Autodesk Inventor part; units mm, degrees
ref_plane "YZ Plane" through (0, 0, 0) normal (1, 0, 0) x (0, 1, 0)
ref_plane "XZ Plane" through (0, 0, 0) normal (0, 1, 0) x (-1, 0, 0)
ref_plane "XY Plane" through (0, 0, 0) normal (0, 0, 1) x (1, 0, 0)
sketch "Sketch1" plane through (0, 0, 0) normal (0, 0, 1) x (1, 0, 0)
  line L0 (0, 0) -> (0, 25.4)
  line L1 (0, 0) -> (25.4, 0)
  line L2 (4.7625, 20.6375) -> (4.7625, 9.525)
  line L3 (9.525, 4.7625) -> (20.6375, 4.7625)
  arc A0 (4.7625, 20.6375) -> (0, 25.4) centre (0, 20.6375) ccw
  arc A1 (25.4, 0) -> (20.6375, 4.7625) centre (20.6375, 0) ccw
  arc A2 (4.7625, 9.525) -> (9.525, 4.7625) centre (9.525, 9.525) ccw
  dimension "d0" = 25.4
  dimension "d1" = 25.4
  dimension "d2" = 4.7625
  dimension "d3" = 4.7625
extrude "Extrusion1" add sketch "Sketch1" along normal blind 25.4
sketch "Sketch2" plane through (0, 0, 0) normal (0, -1, 0) x (1, 0, 0)
  line L0 (25.4, 25.4) -> (0, 25.4)
  line L1 (25.4, 0) -> (25.4, 25.4)
  circle A0 centre (12.7, 12.7) radius 3.175
  dimension "d6" = 6.35
  dimension "d7" = 12.7
  dimension "d8" = 12.7
extrude "Extrusion2" cut sketch "Sketch2" against normal blind 25.4
sketch "Sketch3" plane through (0, 0, 0) normal (-1, 0, 0) x (0, 0, 1)
  circle A0 centre (12.7, 12.7) radius 3.175
  dimension "d11" = 6.35
extrude "Extrusion3" cut sketch "Sketch3" against normal blind 25.4
equation "\"d3\" = d2"
properties part number "small L bracket"
The model under review builds one solid part; all positions refer to its coordinate system, in mm. A direction names the side the tool comes from. Coordinates: 2 decimals unless noted, no trailing zeros. Write each loop counter-clockwise with the first axis right and the second up, starting at its lowest first coordinate (ties: lowest second). Pieces come first, ordered by that corner, then holes.
1) We need section A-A on y = 12.7. State the section outline as (x, z) points (1 decimal), then the cut area to 3 significant figures.
2) We need section D-D on x = 3. State the section outline as (y, z) points (3 decimals), then the cut area to 3 significant figures.
3) Machinability: for faces 4 (the face through (10.18, 2.35, 10.77)), 5 (the face through (16.2, 4.762, 12.5)), which of the approach directions +Z, -Z, +X, -X, +Y, -Y give a long, thin tool a straight path to every point of the face, cutting with its end or side? Answer none if there is none.
4) We need section C-C on z = 8.5. State the section outline as (x, y) points (1 decimal), then the cut area to 3 significant figures.
5) The part is to be moulded in two halves that separate along Z. For faces 1 (the face through (0, 15.3, 15.3)), 2 (the face through (2.35, 10.77, 10.18)), 3 (the face through (4, 7, 25.4)), say which applies: pulls with the +Z half, pulls with the -Z half, needs draft (parallel to the pull), parting line crosses it, or undercut.
6) To check wall thickness, follow probe 1 along Z at (x, y) = (1.75, 12.7) (3 decimals); probe 2 along Y at (x, z) = (20, 11). State the ranges of each line that lie inside material, in increasing order.
7) Clearance check with flat-ended pins moving along their axes: pin 1 Ø5 at (x, z) = (9, 14.5) entering from +Y; pin 2 Ø12 at (y, z) = (15, 14.5) entering from +X; pin 3 Ø5 at (x, z) = (12.7, 12.7) entering from +Y; pin 4 Ø12 at (x, z) = (13, 17.5) entering from +Y. State where each tip first meets the part, or that it passes through.
Answer list:
1. outline: (0, 0) - (4.8, 0) - (4.8, 9.5) - (0, 9.5) - close; (0, 15.9) - (4.8, 15.9) - (4.8, 25.4) - (0, 25.4) - close
1. area: 90.7 mm2
2. outline: (0, 0) - (24.336, 0) - (24.336, 25.4) - (0, 25.4) - close; hole circle Ø6.35 at (12.7, 12.7)
2. area: 586 mm2
3. face 4: +Y, -Y
3. face 5: +Z, -Z, +X, +Y
4. outline: (0, 0) - (25.4, 0) arc R4.8 ccw to (20.6, 4.8) - (9.5, 4.8) arc R4.8 cw to (4.8, 9.5) - (4.8, 20.6) arc R4.8 ccw to (0, 25.4) - close
4. area: 214 mm2
5. face 1: needs draft
5. face 2: undercut
5. face 3: pulls with the +Z half
6. probe 1: z = 0 to 9.525, 15.875 to 25.4
6. probe 2: y = 0 to 4.76
7. pin 1: stops at y = 5.85
7. pin 2: stops at x = 4.79
7. pin 3: passes through
7. pin 4: stops at y = 5.49
